from build123d import *

# Parameters (mm, degrees)
SKETCH_1_R          = 1.4
EXTRUDE_1_DEPTH     = 1.4
SKETCH_2_R          = 0.7
EXTRUDE_2_DEPTH     = 10
CUT_EXTRUDE_1_DEPTH = 1
SKETCH_4_R          = 2.875018911
CUT_EXTRUDE_2_DEPTH = 4


with BuildPart() as part:
    # 草图1 → 凸台-拉伸1 (new body)
    with BuildSketch(Plane.XY):
        Circle(SKETCH_1_R)
    extrude(amount=EXTRUDE_1_DEPTH)

    # 草图2 → 凸台-拉伸2 (add)
    with BuildSketch(Plane.XY.offset(1.4)):
        Circle(SKETCH_2_R)
    extrude(amount=EXTRUDE_2_DEPTH)

    # 草图3 → 切除-拉伸1 (cut)
    with BuildSketch(Plane(origin=(0, 0, 0), x_dir=(-1, 0, 0), z_dir=(0, 0, -1))):
        Polygon((0, 0.68), (-0.588897275, 0.34), (-0.588897275, -0.34), (0, -0.68), (0.588897275, -0.34), (0.588897275, 0.34), align=None)
    extrude(amount=-CUT_EXTRUDE_1_DEPTH, mode=Mode.SUBTRACT)

    # 草图4 → 切除-拉伸2 (cut)
    with BuildSketch(Plane.XY.offset(11.4)):
        Circle(SKETCH_4_R)
    extrude(amount=-CUT_EXTRUDE_2_DEPTH, mode=Mode.SUBTRACT)


solid = part.part
The model under review builds one solid part; all positions refer to its coordinate system, in mm. A direction names the side the tool comes from. Round coordinates to 2 decimals unless told otherwise and drop trailing zeros. Loops run counter-clockwise (first coordinate to the right, second up) from the corner with the lowest first, then second, coordinate; pieces in that order, holes last. Notation, with made-up numbers: (76, -12.75) -> (113, -12.75) arc R20 cw to (113, 23.25) -> close; hole circle Ø10 at (45.5, 30.5). An arc over 180 degrees is marked (long way). Write item = value, one per line. Start each with the question number.
Item 1: Take a section at A-A on y = 0. Give the boundary of the cut face in (x, z).
Item 2: To check wall thickness, follow L1, parallel to Z at x = -0.3, y = -0.7; L2, parallel to Y at x = 0.3, z = 0.5; L3, parallel to X at y = 0.05, z = 6.5. State the ranges of each line that lie inside material, in increasing order.
Item 3: Take a section at D-D on x = -1.1. Give the boundary of the cut face in (y, z).
Item 4: For faces 1 (the cylindrical face through (-0.7, 0, 4.4)), 2 (the flat face through (1, 0, 0)), list the 3-axis set-ups (+Z, -Z, +X, -X, +Y, -Y) from which the entire face can be reached by the end or side of a thin tool; tool diameter is ignored.
Item 5: Mouldability with a two-part tool opening along X and no side actions: class faces 3 (the cylindrical face through (-1.4, 0.06, 0.69)), 4 (the flat face through (0, 0, 7.4)), 5 (the flat face through (0, 0, 1)) as released by +X, released by -X, zero draft, split by the parting line, or undercut.
Item 6: Insertion check: pin 1 (1.5 mm diameter, centred on x = 1, y = 0, fed in from -Z). The pin has a flat end and moves straight along its axis. Give the tip position at first contact, or say it passes through.
Item 7: Take a section at C-C on z = 4.75. Give the boundary of the cut face in (x, y).
Item 8: Take a section at B-B on x = -0.4. Give the boundary of the cut face in (y, z).
Result:
q1.outline = (-1.4, 0) -> (-0.59, 0) -> (-0.59, 1) -> (0.59, 1) -> (0.59, 0) -> (1.4, 0) -> (1.4, 1.4) -> (0.7, 1.4) -> (0.7, 7.4) -> (-0.7, 7.4) -> (-0.7, 1.4) -> (-1.4, 1.4) -> close
q2.L1 = 0 to 1.4
q2.L2 = -1.37 to -0.51, 0.51 to 1.37
q2.L3 = -0.7 to 0.7
q3.outline = (-0.87, 0) -> (0.87, 0) -> (0.87, 1.4) -> (-0.87, 1.4) -> close
q4.face_1 = +Z
q4.face_2 = -Z, +X, -X, +Y, -Y
q5.face_3 = split by the parting line
q5.face_4 = zero draft
q5.face_5 = undercut
q6.pin_1 = 0
q7.outline = circle Ø1.4 at (0, 0)
q8.outline = (-1.34, 0) -> (-0.45, 0) -> (-0.45, 1) -> (0.45, 1) -> (0.45, 0) -> (1.34, 0) -> (1.34, 1.4) -> (0.57, 1.4) -> (0.57, 7.4) -> (-0.57, 7.4) -> (-0.57, 1.4) -> (-1.34, 1.4) -> close
